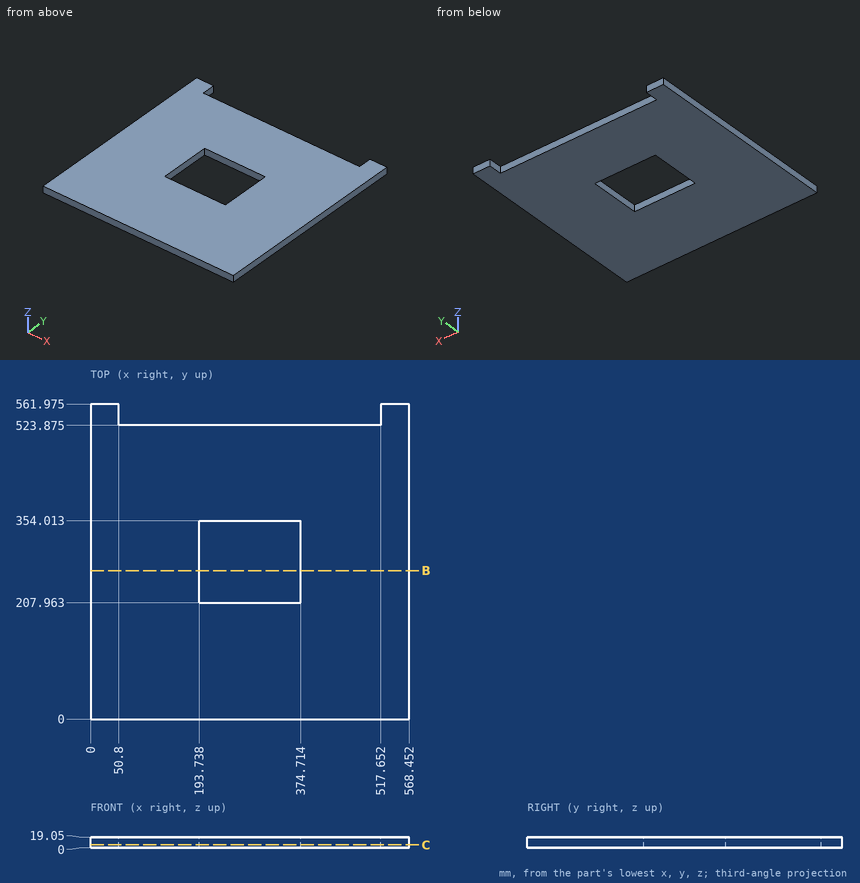
Verification items for this drawing (mm, ordinates from the low corner). Give positions to 0.01 mm unless a question says otherwise; leave off trailing zeros. Write each loop counter-clockwise with the first axis right and the second up, starting at its lowest first coordinate (ties: lowest second). Pieces come first, ordered by that corner, then holes.
1) Thickness scan on line 1 (Y direction, x = 225, z = 12.5) (1 decimal); line 2 (X direction, y = 297, z = 1.5); line 3 (X direction, y = 536, z = 10.5). Record the ranges inside material, lowest first.
Values follow:
line 1: y = 0 to 208, 354 to 523.9
line 2: x = 0 to 193.74, 374.71 to 568.45
line 3: x = 0 to 50.8, 517.65 to 568.45
2) Cross-section at C-C (z = 5.5). Record the boundary of the cut face in (x, y) (1 decimal).
Values follow:
outline: (0, 0) - (568.5, 0) - (568.5, 562) - (517.7, 562) - (517.7, 523.9) - (50.8, 523.9) - (50.8, 562) - (0, 562) - close; hole (193.7, 208) - (374.7, 208) - (374.7, 354) - (193.7, 354) - close
3) Go/stop test with a flat-tipped pin: pin 1 Ø5.5 at (x, z) = (242.5, 10) entering from +Y (1 decimal). Record where the tip stops, or that it passes through.
Values follow:
pin 1: stops at y = 523.9
4) Cross-section at B-B (y = 265). Record the boundary of the cut face in (x, z), plus the area to 3 significant figures.
Values follow:
outline: (0, 0) - (193.74, 0) - (193.74, 19.05) - (0, 19.05) - close; (374.71, 0) - (568.45, 0) - (568.45, 19.05) - (374.71, 19.05) - close
area: 7,380 mm2
